Check sheet for the modelled part. Datum: model origin and axes. Units: mm. A direction names the side the tool comes from. Round coordinates to 2 decimals unless told otherwise and drop trailing zeros. Write each loop counter-clockwise with the first axis right and the second up, starting at its lowest first coordinate (ties: lowest second). Pieces come first, ordered by that corner, then holes. Notation, with made-up numbers: M 83,60.5 L 133,60.5 A31 cw 133,97.5 Z; hole C 20,69 d11. An arc over 180 degrees is marked long. Put each result on its own line as item: value.
```python
from build123d import *

# Parameters (mm, degrees)
SKETCH1_R           = 2.375
EXTRUDE1_DEPTH      = 10
SHELL1_T            = -0.2
SKETCH2_R           = 0.05
EXTRUDE2_DEPTH      = 9.65
EXTRUDE2_DEPTH_BACK = 9.65
SKETCH7_R           = 2.55
EXTRUDE6_DEPTH      = 5
FILLET2_R           = 0.25
SKETCH8_R           = 2.55
EXTRUDE7_DEPTH      = 5
FILLET3_R           = 0.25


with BuildPart() as part:
    # Sketch1 → Extrude1 (new, symmetric)
    with BuildSketch(Plane(origin=(0, 0, 0), x_dir=(0, 0, -1), z_dir=(1, 0, 0))):
        Circle(SKETCH1_R)
    extrude(amount=EXTRUDE1_DEPTH, both=True)

    # Shell1
    shell1_openings = [part.faces().sort_by_distance(p)[0] for p in [
        (10, 0, 0),
        (-10, 0, 0),
    ]]
    offset(amount=SHELL1_T, openings=shell1_openings, kind=Kind.INTERSECTION)



with BuildPart() as body_2:
    # Sketch2 → Extrude2 (new, two sides)
    with BuildSketch(Plane(origin=(0, 0, 0), x_dir=(0, 0, -1), z_dir=(1, 0, 0))) as extrude2_sk:
        Circle(SKETCH2_R)
    extrude(amount=EXTRUDE2_DEPTH)
    extrude(extrude2_sk.sketch, amount=-EXTRUDE2_DEPTH_BACK)


with BuildPart() as part_1:
    add(part.part)

    add(body_2.part)  # Extrude6 merges body 2
    # Sketch7 → Extrude6 (add)
    with BuildSketch(Plane(origin=(10.5, 0, 0), x_dir=(0, 0, -1), z_dir=(1, 0, 0))):
        Circle(SKETCH7_R)
    extrude(amount=-EXTRUDE6_DEPTH)

    # Fillet2
    fillet2_edges = [part_1.edges().sort_by_distance(p)[0] for p in [
        (10.5, 0, 2.55),
    ]]
    fillet(fillet2_edges, radius=FILLET2_R)

    # Sketch8 → Extrude7 (add)
    with BuildSketch(Plane.ZY.offset(10.5)):
        with Locations(Location((0, 0, 0), (0, 0, 180))):
            Circle(SKETCH8_R)
    extrude(amount=-EXTRUDE7_DEPTH)

    # Fillet3
    fillet3_edges = [part_1.edges().sort_by_distance(p)[0] for p in [
        (-10.5, 0, 2.55),
    ]]
    fillet(fillet3_edges, radius=FILLET3_R)


solid = part_1.part
```
1. Access from +Z, -Z, +X, -X, +Y, -Y to the whole of each face (thin tool, end or side, straight path). Record for faces 1 (the cylindrical face through (0.077, -2.123, 0.471)), 2 (the cylindrical face through (-7.91, -0.77, -2.43)).
Computed values:
face 1: none
face 2: +X, -X
2. Depth check by flat-ended pin: pin 1 Ø3 at (x, y) = (-1.5, 0) entering from +Z (3 decimals). Enter the tip coordinate at first touch or a pass-through.
Computed values:
pin 1: stops at z = 2.375
3. Scan lines: probe 1 along X at (y, z) = (1.1, 1.4); probe 2 along Y at (x, z) = (-2.75, 0.1); probe 3 along X at (y, z) = (1.65, -1.65). Record each from-to range of solid material in increasing order.
Computed values:
probe 1: x = -10.5 to -5.5, 5.5 to 10.5
probe 2: y = -2.37 to -2.17, 2.17 to 2.37
probe 3: x = -10.5 to 10.5
4. Cross-section at B-B (x = -8). Enter the section's corners in (y, z).
Computed values:
outline: C 0,0 d5.1
5. Cross-section at A-A (x = -4). Enter the section's corners in (y, z) (3 decimals).
Computed values:
outline: C 0,0 d4.75; C 0,0 d0.1; hole C 0,0 d4.35
6. Release check for a two-part mould opening along X. For faces 3 (the flat face through (10.5, 0, 0)), 4 (the cylindrical face through (7.91, -2.26, -1.18)), 5 (the cylindrical face through (0.077, -2.107, -1.096)) record: +X half, -X half, draft (parallel to the pull), parting line (faces both ways), or undercut.
Computed values:
face 3: +X half
face 4: draft
face 5: undercut
